Autodesk Inventor part; units mm, degrees
ref_plane "YZ Plane" through (0, 0, 0) normal (1, 0, 0) x (0, 1, 0)
ref_plane "XZ Plane" through (0, 0, 0) normal (0, 1, 0) x (-1, 0, 0)
ref_plane "XY Plane" through (0, 0, 0) normal (0, 0, 1) x (1, 0, 0)
sketch "Sketch1" plane through (0, 0, 0) normal (0, 0, 1) x (1, 0, 0)
  line L0 (16, -32) -> (-16, -32)
  line L1 (-16, -32) -> (-16, 32)
  line L2 (-16, 32) -> (16, 32)
  line L3 (16, 32) -> (16, -32)
  line L4 (16, -32) -> (-16, 32) construction
  line L5 (-16, -32) -> (16, 32) construction
  circle A0 centre (0, -22) radius 2.5 construction
  circle A1 centre (-6, -28) radius 2
  circle A2 centre (6, -28) radius 2
  circle A3 centre (6, -16) radius 2
  circle A4 centre (-6, -16) radius 2
  line L6 (-16, 0) -> (16, 0) construction
  point P0 (0, 0)
  point P1 (0, -32)
  dimension "d0" = 32
  dimension "d1" = 64
  dimension "d2" = 5
  dimension "d3" = 10
  dimension "d4" = 4
  dimension "d5" = 6
  dimension "d6" = 6
  dimension "d9" = 360
extrude "Extrusion1" add sketch "Sketch1" along normal mid plane 3.175
sketch "Sketch2" plane through (0, 0, 1.5875) normal (0, 0, 1) x (1, 0, 0)
  line L0 (16, 32) -> (-16, 32) construction
  line L1 (-16, 32) -> (-16, -32) construction
  line L2 (-16, -32) -> (16, -32) construction
  line L3 (16, -32) -> (16, 32) construction
  circle A0 centre (-6, -16) radius 2 construction
  circle A1 centre (6, -16) radius 2 construction
  circle A2 centre (6, -28) radius 2 construction
  circle A3 centre (-6, -28) radius 2 construction
  circle A4 centre (0, 20) radius 7
  circle A5 centre (-12, 28) radius 2
  line L4 (0, 32) -> (0, -32) construction
  line L5 (-16, 32) -> (-16, -32)
  line L6 (-16, 0) -> (16, 0) construction
  circle A6 centre (-12, 12) radius 2
  circle A7 centre (-12, -4) radius 2
  circle A8 centre (12, 28) radius 2
  circle A9 centre (12, 12) radius 2
  circle A10 centre (12, -4) radius 2
  point P0 (0, 0)
  dimension "d14" = 14
  dimension "d15" = 20
  dimension "d16" = 4
  dimension "d17" = 4
  dimension "d18" = 4
  dimension "d19" = 4
  dimension "d20" = 16
  dimension "d21" = 4
  dimension "d22" = 16
extrude "Extrusion2" cut sketch "Sketch2" against normal through all
chamfer "Chamfer1" distance 2 angle 45 4 edges at (16, 32, 0) (-16, 32, 0) (16, -32, 0) (-16, -32, 0)
properties part number "ArmSidePlate"
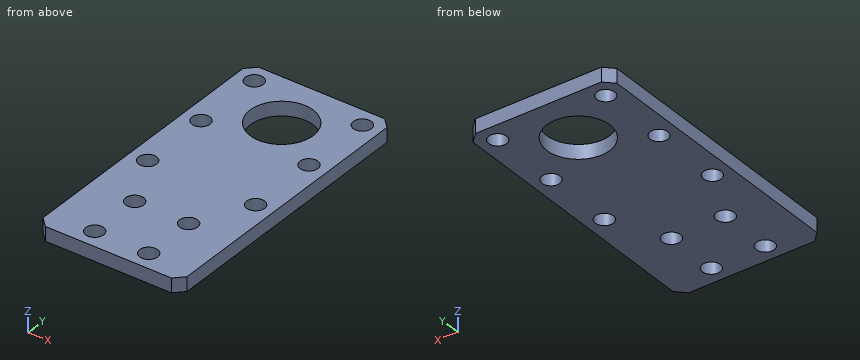
Could you check a few things on this model? Use its own coordinates, in mm. Coordinates: 2 decimals unless noted, no trailing zeros. Write each loop counter-clockwise with the first axis right and the second up, starting at its lowest first coordinate (ties: lowest second). Pieces come first, ordered by that corner, then holes. Notation, with made-up numbers: (50.5, -14) - (58.5, -14) arc R9 cw to (58.5, 0) - close; hole circle Ø9 at (-29.75, 0.25). An arc over 180 degrees is marked (long way). Write item = value, one per line.
1) Suppose I cut it at B-B on y = -16. Please give me the cut outline in (x, z), plus the area to 3 significant figures.
Result set:
outline = (-16, -1.59) - (-8, -1.59) - (-8, 1.59) - (-16, 1.59) - close; (-4, -1.59) - (4, -1.59) - (4, 1.59) - (-4, 1.59) - close; (8, -1.59) - (16, -1.59) - (16, 1.59) - (8, 1.59) - close
area = 76.2 mm2
2) Please list where these lines run through material, in increasing order: line 1 (Y direction, x = 12, z = -0.9); line 2 (X direction, y = -17, z = 1.3); line 3 (Y direction, x = -6, z = -0.6). Write a range as [from, to].
Result set:
line_1 = [-32, -6], [-2, 10], [14, 26], [30, 32]
line_2 = [-16, -7.73], [-4.27, 4.27], [7.73, 16]
line_3 = [-32, -30], [-26, -18], [-14, 16.39], [23.61, 32]
3) Suppose I cut it at D-D on z = 0.1. State how many separate pieces and enclosed holes the cut face has, plus the area to 3 significant figures.
Result set:
separate_pieces = 1
enclosed_holes = 11
area = 1,760 mm2
4) Suppose I cut it at C-C on x = 0. Please give me the cut outline in (y, z), plus the area to 3 significant figures.
Result set:
outline = (-32, -1.59) - (13, -1.59) - (13, 1.59) - (-32, 1.59) - close; (27, -1.59) - (32, -1.59) - (32, 1.59) - (27, 1.59) - close
area = 159 mm2
5) Suppose I cut it at A-A on x = 12. Please give me the cut outline in (y, z).
Result set:
outline = (-32, -1.59) - (-6, -1.59) - (-6, 1.59) - (-32, 1.59) - close; (-2, -1.59) - (10, -1.59) - (10, 1.59) - (-2, 1.59) - close; (14, -1.59) - (26, -1.59) - (26, 1.59) - (14, 1.59) - close; (30, -1.59) - (32, -1.59) - (32, 1.59) - (30, 1.59) - close
